Check sheet for the modelled part. Datum: model origin and axes. Units: mm. A direction names the side the tool comes from. Give positions to 0.01 mm unless a question says otherwise; leave off trailing zeros. Order: outer loops, then holes, each group sorted by start corner. A loop starts at its lowest first (then second) coordinate and runs counter-clockwise, first axis right, second up. Notation, with made-up numbers: (-3, -9.5) - (37, -9.5) arc R25 ccw to (37, 14.5) - close; hole circle Ø5 at (36, 59). An arc over 180 degrees is marked (long way). Answer in a Markdown table with one row per item.
from build123d import *

# Parameters (mm, degrees)
BOSS_EXTRUDE1_DEPTH    = 5
M4_CLEARANCE_HOLE1_D   = 4.5
FILLET1_R              = 3
M1_6_CLEARANCE_HOLE1_D = 1.8


with BuildPart() as part:
    # Sketch2 → Boss-Extrude1 (new body)
    with BuildSketch(Plane.XY):
        Polygon((11.25, 46.75), (-6.25, 46.75), (-6.25, 11.25), (6.25, 11.25), (6.25, -11.25), (-6.25, -11.25), (-6.25, -37.25), (11.25, -37.25), align=None)
    extrude(amount=BOSS_EXTRUDE1_DEPTH)

    # M4 Clearance Hole1 (through all)
    with Locations(Plane(origin=(0, 0, 0), x_dir=(1, 0, 0), z_dir=(0, 0, -1))):
        with Locations((0, -39.25), (0, 29.75)):
            Hole(M4_CLEARANCE_HOLE1_D / 2)

    # Fillet1
    fillet1_edges = [part.edges().sort_by_distance(p)[0] for p in [
        (-6.25, 46.75, 2.5),
        (11.25, 46.75, 2.5),
        (11.25, -37.25, 2.5),
        (-6.25, -37.25, 2.5),
    ]]
    fillet(fillet1_edges, radius=FILLET1_R)

    # M1.6 Clearance Hole1 (through all)
    with Locations(Plane(origin=(0, 0, 0), x_dir=(1, 0, 0), z_dir=(0, 0, -1))):
        with Locations((0, -13.5), (0, 13.5)):
            Hole(M1_6_CLEARANCE_HOLE1_D / 2)


solid = part.part
(1) Thickness scan on L1, parallel to Y at x = 0, z = 3.9; L2, parallel to X at y = -13.5, z = 2; L3, parallel to Y at x = 1.25, z = 0.9. Record the ranges inside material, lowest first.
Geometry says:
| item | result |
|---|---|
| L1 | -37.25 to -32, -27.5 to -14.4, -12.6 to -11.25, 11.25 to 12.6, 14.4 to 37, 41.5 to 46.75 |
| L2 | -6.25 to -0.9, 0.9 to 11.25 |
| L3 | -37.25 to -31.62, -27.88 to -11.25, 11.25 to 37.38, 41.12 to 46.75 |
(2) Cross-section at B-B, the plane x = 0. Record the cut outline in (y, z), then the cut area to 4 significant figures.
Geometry says:
| item | result |
|---|---|
| outline | (-37.25, 0) - (-32, 0) - (-32, 5) - (-37.25, 5) - close; (-27.5, 0) - (-14.4, 0) - (-14.4, 5) - (-27.5, 5) - close; (-12.6, 0) - (-11.25, 0) - (-11.25, 5) - (-12.6, 5) - close; (11.25, 0) - (12.6, 0) - (12.6, 5) - (11.25, 5) - close; (14.4, 0) - (37, 0) - (37, 5) - (14.4, 5) - close; (41.5, 0) - (46.75, 0) - (46.75, 5) - (41.5, 5) - close |
| area | 244.5 mm² |
(3) Cross-section at C-C, the plane z = 1.15. Record the cut outline in (x, y), then the cut area to 3 significant figures.
Geometry says:
| item | result |
|---|---|
| outline | (-6.25, -34.25) arc R3 ccw to (-3.25, -37.25) - (8.25, -37.25) arc R3 ccw to (11.25, -34.25) - (11.25, 43.75) arc R3 ccw to (8.25, 46.75) - (-3.25, 46.75) arc R3 ccw to (-6.25, 43.75) - (-6.25, 11.25) - (6.25, 11.25) - (6.25, -11.25) - (-6.25, -11.25) - close; hole circle Ø4.5 at (0, -29.75); hole circle Ø4.5 at (0, 39.25); hole circle Ø1.8 at (0, -13.5); hole circle Ø1.8 at (0, 13.5) |
| area | 1,140 mm² |
(4) Access from +Z, -Z, +X, -X, +Y, -Y to the whole of each face (thin tool, end or side, straight path). Record for faces 5 (the flat face through (-6.25, 28, 2)), 6 (the flat face through (6.25, 0, 2)).
Geometry says:
| item | result |
|---|---|
| face 5 | +Z, -Z, -X, +Y, -Y |
| face 6 | +Z, -Z, -X |
(5) Cross-section at D-D, the plane x = 5. Record the cut outline in (y, z), then the cut area to 4 significant figures.
Geometry says:
| item | result |
|---|---|
| outline | (-37.25, 0) - (-11.25, 0) - (-11.25, 5) - (-37.25, 5) - close; (11.25, 0) - (46.75, 0) - (46.75, 5) - (11.25, 5) - close |
| area | 307.5 mm² |
(6) Cross-section at A-A, the plane y = -13.5. Record the cut outline in (x, z).
Geometry says:
| item | result |
|---|---|
| outline | (-6.25, 0) - (-0.9, 0) - (-0.9, 5) - (-6.25, 5) - close; (0.9, 0) - (11.25, 0) - (11.25, 5) - (0.9, 5) - close |
(7) Gauge pin test, flat ends, axial feed: P1, Ø2.5, axis at y = -3, z = 3.5, coming from the -X side; P2, Ø6, axis at x = 0, y = -29.75, coming from the -Z side. Record the tip position at first contact, or that the pin passes through.
Geometry says:
| item | result |
|---|---|
| P1 | x = 6.25 |
| P2 | z = 0 |
(8) Mould release check, pull along Y, two halves, no side actions. Record for faces 1 (the flat face through (0, 11.25, 2)), 2 (the cylindrical face through (-5.35, -36.39, 2.54)), 3 (the flat face through (0, -11.25, 2)), 4 (the flat face through (3, 46.75, 2)): pulls with the +Y half, pulls with the -Y half, needs draft (parallel to the pull), parting line crosses it, or undercut.
Geometry says:
| item | result |
|---|---|
| face 1 | undercut |
| face 2 | pulls with the -Y half |
| face 3 | undercut |
| face 4 | pulls with the +Y half |
